```python
from build123d import *

# Parameters (mm, degrees)
SKETCH1_W          = 25.4
SKETCH1_H          = 152.4
SKETCH2_W          = 19.05
SKETCH2_H          = 114.3
CUT_REVOLVE1_ANGLE = 120


with BuildPart() as part:
    # Sketch1 → Revolve1 (revolve)
    with BuildSketch(Plane.XY):
        with Locations((76.2, 76.2)):
            Rectangle(SKETCH1_W, SKETCH1_H)
    revolve(axis=Axis((0, 0, 0), (0, 1, 0)))

    # Sketch2 → Cut-Revolve1 (revolve, cut)
    with BuildSketch(Plane.XY):
        with Locations((79.375, 69.85)):
            Rectangle(SKETCH2_W, SKETCH2_H)
    revolve(axis=Axis((0, 0, 0), (0, 1, 0)), revolution_arc=CUT_REVOLVE1_ANGLE, mode=Mode.SUBTRACT)


solid = part.part
```
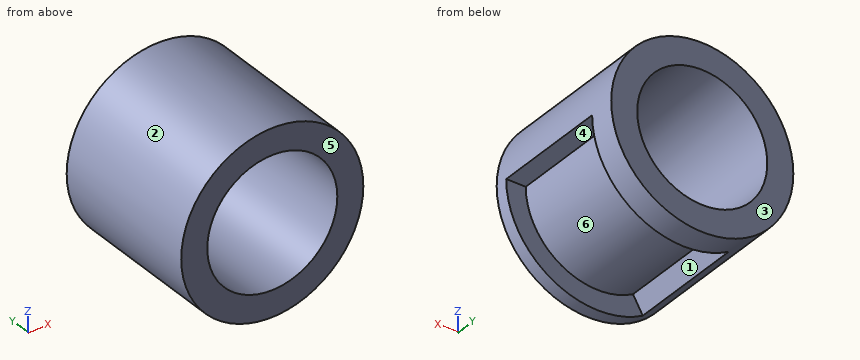
For this review, take the finished solid that the model builds, in its own axes (mm). Face numbers are marked on the shaded views. A direction names the side the tool comes from. Coordinates: 2 decimals unless noted, no trailing zeros. Order: outer loops, then holes, each group sorted by start corner. A loop starts at its lowest first (then second) coordinate and runs counter-clockwise, first axis right, second up. Notation, with made-up numbers: (23, 43) - (55, 43) arc R24 ccw to (55, 75) - close; hole circle Ø5 at (58, 49.5). An arc over 180 degrees is marked (long way). Answer as a JSON object with one key per item and string values. Group by question number.
1. Clearance check with flat-ended pins moving along their axes: P1, Ø2, axis at x = -20.5, y = 30, coming from the -Z side; P2, Ø12, axis at y = 64.5, z = -12.5, coming from the +X side; P3, Ø1, axis at x = -47.5, y = 60, coming from the -Z side. State where each tip first meets the part, or that it passes through.
2. We need section C-C on y = 120.5. State the section outline as (x, z) points (3 decimals).
3. For the marked faces 4, 5 and 6, list the 3-axis set-ups (+Z, -Z, +X, -X, +Y, -Y) from which the entire face can be reached by the end or side of a thin tool; tool diameter is ignored.
4. For probe 1 along Z at (x, y) = (0, 40.5); probe 2 along Y at (x, z) = (11.5, -79.5); probe 3 along Z at (x, y) = (14.5, 82), list the stretches that pass through material, from the lowest coordinate up.
5. We need section B-B on z = -23.5. State the section outline as (x, y) points, then the cut area to 3 significant figures.
6. We need section A-A on x = 0. State the section outline as (y, z) points, then the cut area to 3 significant figures.
7. We need section D-D on z = 46. State the section outline as (x, y) points (3 decimals).
8. The part is to be moulded in two halves that separate along X. For the marked faces 1, 2 and 3, say which applies: pulls with the +X half, pulls with the -X half, needs draft (parallel to the pull), parting line crosses it, or undercut.
Final values:
{
 "1": {"P1": "z = -67.07", "P2": "x = 69.55", "P3": "z = -75.46"},
 "2": {"outline": "(-44.45, -76.99) - (-34.925, -60.492) arc R69.85 ccw to (69.85, 0) - (88.9, 0) arc R88.9 ccw (long way) to start; hole circle Ø127 at (0, 0)"},
 "3": {"face 4": "-Z, +X", "face 5": "+Z, -Z, +X, -X, -Y", "face 6": "-Z"},
 "4": {"probe 1": "-69.85 to -63.5, 63.5 to 88.9", "probe 2": "0 to 12.7, 127 to 152.4", "probe 3": "-68.33 to -61.82, 61.82 to 87.71"},
 "5": {"outline": "(-85.74, 0) - (-58.99, 0) - (-58.99, 152.4) - (-85.74, 152.4) - close; (58.99, 0) - (85.74, 0) - (85.74, 12.7) - (65.78, 12.7) - (65.78, 127) - (85.74, 127) - (85.74, 152.4) - (58.99, 152.4) - close", "area": "5,870 mm²"},
 "6": {"outline": "(0, -88.9) - (12.7, -88.9) - (12.7, -69.85) - (127, -69.85) - (127, -88.9) - (152.4, -88.9) - (152.4, -63.5) - (0, -63.5) - close; (0, 63.5) - (152.4, 63.5) - (152.4, 88.9) - (0, 88.9) - close", "area": "5,560 mm²"},
 "7": {"outline": "(-76.074, 0) - (-43.775, 0) - (-43.775, 152.4) - (-76.074, 152.4) - close; (43.775, 0) - (76.074, 0) - (76.074, 152.4) - (43.775, 152.4) - close"},
 "8": {"face 1": "undercut", "face 2": "parting line crosses it", "face 3": "needs draft"}
}
